The listing builds one solid part. Answer for the finished solid, in the listing's coordinates (mm). Coordinates: 2 decimals unless noted, no trailing zeros. Write each loop counter-clockwise with the first axis right and the second up, starting at its lowest first coordinate (ties: lowest second). Pieces come first, ordered by that corner, then holes. Notation, with made-up numbers: M 52.5,-26.5 L 102.5,-26.5 A26 ccw 102.5,5.5 Z; hole C 72,88.25 d10. An arc over 180 degrees is marked long. Put each result on its own line as item: value. Start each with the question number.
```python
from build123d import *

# Parameters (mm, degrees)
SKETCH1_R           = 22
SKETCH1_R_2         = 12.5
BOSS_EXTRUDE1_DEPTH = 15
CHAMFER1_SIZE       = 1
CHAMFER2_SIZE       = 5
CHAMFER2_SIZE2      = 10
CHAMFER3_SIZE       = 10
CHAMFER3_SIZE2      = 5


with BuildPart() as part:
    # Sketch1 → Boss-Extrude1 (new, symmetric)
    with BuildSketch(Plane.XY):
        Circle(SKETCH1_R)
        Circle(SKETCH1_R_2, mode=Mode.SUBTRACT)
    extrude(amount=BOSS_EXTRUDE1_DEPTH, both=True)

    # Chamfer1
    chamfer1_edges = [part.edges().sort_by_distance(p)[0] for p in [
        (-22, 0, -15),
        (-22, 0, 15),
    ]]
    chamfer(chamfer1_edges, length=CHAMFER1_SIZE)

    # Chamfer2
    chamfer2_edges = [part.edges().sort_by_distance(p)[0] for p in [
        (-12.5, 0, 15),
    ]]
    chamfer2_side = [part.faces().sort_by_distance(p)[0] for p in [
        (-20.406030304, 0, 15),
    ]]
    chamfer(chamfer2_edges, length=CHAMFER2_SIZE, length2=CHAMFER2_SIZE2, reference=chamfer2_side[0])

    # Chamfer3
    chamfer3_edges = [part.edges().sort_by_distance(p)[0] for p in [
        (-12.5, 0, -15),
    ]]
    chamfer3_side = [part.faces().sort_by_distance(p)[0] for p in [
        (-12.5, 0, -5),
    ]]
    chamfer(chamfer3_edges, length=CHAMFER3_SIZE, length2=CHAMFER3_SIZE2, reference=chamfer3_side[0])


solid = part.part
```
1) Straight lines are drawn through the part: probe 1 along Y at (x, z) = (0, -1.5); probe 2 along Y at (x, z) = (-6, -6); probe 3 along X at (y, z) = (-10.5, 14.5). For each, find the intervals that lie inside material, in ascending order.
2) A cutting plane is placed at C-C on z = -7.5. Write down the section's boundary in (x, y), then the cut area to 3 significant figures.
3) Determine the mould class of faces 1 (the face through (-10.112, -7.754, 5.486)), 2 (the face through (-4.769, -21.477, 0.196)), 3 (the face through (-8, 16, 15)), 4 (the face through (11.923, 3.755, -0.07)) for opening direction Y: +Y half, -Y half, draft (parallel to the pull), parting line (faces both ways), or undercut.
4) Given pin 1 Ø4 at (y, z) = (10, 3.5) entering from +X; pin 2 Ø3 at (x, z) = (-14.5, -3) entering from -Y; pin 3 Ø3 at (x, z) = (7.5, -1) entering from +Y, each flat-ended and moving along its own axis, determine where each tip first touches the part or whether it passes through.
5) A cutting plane is placed at A-A on x = 0. Write down the section's boundary in (y, z), then the cut area to 3 significant figures.
Answers follow:
1. probe 1: y = -22 to -12.5, 12.5 to 22
1. probe 2: y = -21.17 to -11.53, 11.53 to 21.17
1. probe 3: x = -18.76 to -13.69, 13.69 to 18.76
2. outline: C 0,0 d44; hole C 0,0 d27.5
2. area: 927 mm²
3. face 1: undercut
3. face 2: parting line
3. face 3: draft
3. face 4: undercut
4. pin 1: stops at x = 20.49
4. pin 2: stops at y = -17.75
4. pin 3: stops at y = 21.17
5. outline: M -22,-14 L -21,-15 L -17.5,-15 L -12.5,-5 L -12.5,5 L -17.5,15 L -21,15 L -22,14 Z; M 12.5,-5 L 17.5,-15 L 21,-15 L 22,-14 L 22,14 L 21,15 L 17.5,15 L 12.5,5 Z
5. area: 468 mm²
